Autodesk Inventor part; units mm, degrees
ref_plane "YZ Plane" through (0, 0, 0) normal (1, 0, 0) x (0, 1, 0)
ref_plane "XZ Plane" through (0, 0, 0) normal (0, 1, 0) x (-1, 0, 0)
ref_plane "XY Plane" through (0, 0, 0) normal (0, 0, 1) x (1, 0, 0)
sketch "Sketch1" plane through (0, 0, 0) normal (0, 1, 0) x (-1, 0, 0)
  line L0 (0, -74.6125) -> (0, -76.2)
  line L1 (0, -76.2) -> (-1.461, -76.8211)
  line L2 (-70.1269, -106.0104) -> (-75.0953, -94.3226)
  line L3 (0, 0) -> (-12.7, 0)
  line L4 (0, 0) -> (12.7, 0)
  line L5 (-75.0953, -94.3226) -> (-12.7, -67.7988)
  line L6 (-12.7, 0) -> (-12.7, -67.7988)
  line L7 (-70.1269, -106.0104) -> (-65.1585, -117.6982)
  line L8 (-65.1585, -117.6982) -> (12.7, -84.6012)
  line L9 (12.7, -84.6012) -> (12.7, 0)
  circle A0 centre (0, -76.2) radius 1.5875
  dimension "d0" = 76.2
  dimension "d1" = 76.2
  dimension "d2" = 113.03
  dimension "d3" = 12.7
  dimension "d4" = 12.7
  dimension "d5" = 12.7
  dimension "d6" = 12.7
  dimension "d7" = 3.175
extrude "Extrusion1" add sketch "Sketch1" along normal blind 6.35
sketch "Sketch2" plane through (-12.7, 0, 0) normal (0, 0, 1) x (1, 0, 0)
  circle A0 centre (12.7, 3.175) radius 1.5875
  point P0 (12.7, 0)
  dimension "d10" = 3.175
extrude "Extrusion2" cut sketch "Sketch2" against normal blind 19.05
sketch "Sketch3" plane through (65.1585, 0, -117.6982) normal (0.9203001, 0, -0.3912131) x (-0.3912131, 0, -0.9203001)
  circle A0 centre (-12.7, 3.175) radius 1.5875
  point P0 (-82.8269, 0)
  dimension "d13" = 3.175
extrude "Extrusion3" cut sketch "Sketch3" against normal blind 19.05
fillet "Fillet1" radius 6.35 1 edges at (-12.7, 3.175, -84.6012)
fillet "Fillet2" radius 6.35 1 edges at (12.7, 3.175, -67.7988)
fillet "Fillet3" radius 6.35 1 edges at (65.1585, 3.175, -117.6982)
fillet "Fillet4" radius 6.35 1 edges at (75.0953, 3.175, -94.3226)
fillet "Fillet5" radius 6.35 1 edges at (12.7, 3.175, 0)
fillet "Fillet6" radius 6.35 1 edges at (-12.7, 3.175, 0)
sketch "Sketch4" plane through (0, 6.35, 0) normal (0, 1, 0) x (1, 0, 0)
  circle A0 centre (0, 76.2) radius 1.5875
  circle A1 centre (0, 76.2) radius 3.175
  point P0 (0, 0)
  dimension "d22" = 6.35
extrude "Extrusion4" cut sketch "Sketch4" against normal blind 1.5875
sketch "Sketch5" plane through (0, 6.35, 0) normal (0, 1, 0) x (1, 0, 0)
  arc A0 (69.2514, 91.8384) -> (72.6111, 100.1665) centre (66.7672, 97.6823) ccw
  circle A1 centre (66.7672, 97.6823) radius 1.5875
  point P0 (0, 0)
  dimension "d25" = 3.175
extrude "Extrusion5" cut sketch "Sketch5" against normal blind 6.35
sketch "Sketch6" plane through (0, 0, 0) normal (0, -1, 0) x (1, 0, 0)
  circle A0 centre (66.7672, -97.6823) radius 1.5875
  arc A1 (72.6111, -100.1665) -> (69.2514, -91.8384) centre (66.7672, -97.6823) ccw
  circle A2 centre (66.7672, -97.6823) radius 3.175
  point P0 (0, 0)
  dimension "d28" = 6.35
extrude "Extrusion6" cut sketch "Sketch6" against normal blind 1.5875
sketch "Sketch7" plane through (0, 0, 0) normal (0, -1, 0) x (1, 0, 0)
  arc A0 (12.7, -6.35) -> (6.35, 0) centre (6.35, -6.35) ccw
  circle A1 centre (6.35, -6.35) radius 1.5875
  point P0 (0, 0)
  dimension "d31" = 3.175
extrude "Extrusion7" cut sketch "Sketch7" against normal blind 6.35
sketch "Sketch8" plane through (0, 0, 0) normal (0, -1, 0) x (1, 0, 0)
  circle A0 centre (6.35, -6.35) radius 1.5875
  arc A1 (12.7, -6.35) -> (6.35, 0) centre (6.35, -6.35) ccw
  circle A2 centre (6.35, -6.35) radius 3.175
  point P0 (0, 0)
  dimension "d34" = 6.35
extrude "Extrusion8" cut sketch "Sketch8" against normal blind 1.5875
sketch "Sketch9" plane through (0, 3.175, -19.05) normal (0, 0, 1) x (1, 0, 0)
  circle A0 centre (0, 0) radius 1.5875
  point P0 (0, -3.175)
extrude "Extrusion9" cut sketch "Sketch9" against normal blind 31.75
sketch "Sketch10" plane through (52.5952, 3.175, -98.5578) normal (0.9203001, 0, -0.3912131) x (-0.3912131, 0, -0.9203001)
  circle A0 centre (0, 0) radius 1.5875
  point P0 (-70.1269, -3.175)
extrude "Extrusion10" cut sketch "Sketch10" against normal blind 31.75
sketch "Sketch11" plane through (0, 6.35, 0) normal (0, 1, 0) x (1, 0, 0)
  line L0 (-12.7, 80.4006) -> (-12.7, 6.35)
  line L1 (0, 57.15) -> (6.35, 57.15)
  line L2 (6.35, 57.15) -> (6.35, 44.45)
  line L3 (6.35, 44.45) -> (-6.35, 44.45)
  line L4 (-6.35, 44.45) -> (-6.35, 57.15)
  line L5 (-6.35, 57.15) -> (0, 57.15)
  point P0 (0, 0)
  dimension "d41" = 6.35
  dimension "d42" = 12.7
  dimension "d43" = 12.7
  dimension "d44" = 12.7
extrude "Extrusion11" cut sketch "Sketch11" against normal blind 31.75
sketch "Sketch12" plane through (0, 6.35, 0) normal (0, 1, 0) x (1, 0, 0)
  line L0 (72.6111, 100.1665) -> (67.6427, 111.8543)
  line L1 (59.3146, 115.214) -> (-8.8342, 86.2445)
  line L2 (29.2195, 88.621) -> (17.5317, 83.6526)
  line L3 (17.5317, 83.6526) -> (15.0475, 89.4965)
  line L4 (15.0475, 89.4965) -> (26.7353, 94.4649)
  line L5 (26.7353, 94.4649) -> (31.7037, 82.7771)
  line L6 (31.7037, 82.7771) -> (20.0159, 77.8087)
  line L7 (20.0159, 77.8087) -> (17.5317, 83.6526)
  point P0 (0, 0)
  point P1 (70.1269, 106.0104)
  dimension "d47" = 57.15
  dimension "d48" = 6.35
  dimension "d49" = 12.7
  dimension "d50" = 12.7
  dimension "d51" = 12.7
extrude "Extrusion12" cut sketch "Sketch12" against normal blind 31.75 contours L5 L6 L7 L2
sketch "Sketch13" plane through (0, 6.35, 0) normal (0, 1, 0) x (1, 0, 0)
  line L0 (17.5317, 83.6526) -> (29.2195, 88.621)
  line L1 (59.3146, 115.214) -> (-8.8342, 86.2445)
  line L2 (17.5317, 83.6526) -> (15.0475, 89.4965)
  line L3 (15.0475, 89.4965) -> (26.7353, 94.4649)
  line L4 (26.7353, 94.4649) -> (29.2195, 88.621)
  point P0 (0, 0)
  dimension "d54" = 6.35
  dimension "d55" = 12.7
extrude "Extrusion13" cut sketch "Sketch13" against normal blind 31.75
sketch "Sketch14" plane through (6.35, 0, 0) normal (0, 0, 1) x (1, 0, 0)
  circle A0 centre (-6.35, 3.175) radius 1.5875
  circle A1 centre (-6.35, 3.175) radius 2.286
  point P0 (-6.35, 0)
  dimension "d58" = 4.572
extrude "Extrusion14" cut sketch "Sketch14" against normal blind 44.45
sketch "Sketch15" plane through (67.6427, 0, -111.8543) normal (0.9203001, 0, -0.3912131) x (-0.3912131, 0, -0.9203001)
  circle A0 centre (-6.35, 3.175) radius 1.5875
  circle A1 centre (-6.35, 3.175) radius 2.286
  point P0 (-76.4769, 0)
  dimension "d61" = 4.572
extrude "Extrusion15" cut sketch "Sketch15" against normal blind 44.45
sketch "Sketch16" plane through (0, 6.35, 0) normal (0, 1, 0) x (1, 0, 0)
  circle A0 centre (0, 76.2) radius 3.175
  line L0 (59.3146, 115.214) -> (-8.8342, 86.2445)
  arc A1 (-8.8342, 86.2445) -> (-12.7, 80.4006) centre (-6.35, 80.4006) ccw
  line L1 (-12.7, 80.4006) -> (-12.7, 6.35)
  line L2 (-31.4662, 97.6823) -> (-24.3054, 108.171)
  line L3 (-24.3054, 108.171) -> (1.4241, 90.6052)
  line L4 (-31.4662, 97.6823) -> (-38.6269, 87.1936)
  line L5 (-38.6269, 87.1936) -> (-12.7, 69.493)
  line L6 (0, 76.2) -> (-2.6222, 77.9902)
  point P0 (0, 0)
  dimension "d64" = 38.1
  dimension "d65" = 12.7
  dimension "d66" = 12.7
extrude "Extrusion16" add sketch "Sketch16" against normal blind 6.35 contours L0 A1 L1 L5 L4 L2 L3
sketch "Sketch17" plane through (0, 6.35, 0) normal (0, 1, 0) x (1, 0, 0)
  line L0 (-24.3054, 108.171) -> (-38.6269, 87.1936)
  line L1 (-38.6269, 87.1936) -> (-12.7, 69.493)
  line L2 (-31.4662, 97.6823) -> (-23.5996, 92.3117)
  circle A0 centre (-23.5996, 92.3117) radius 1.5875
  point P0 (0, 0)
  dimension "d69" = 9.525
  dimension "d70" = 3.175
extrude "Extrusion17" cut sketch "Sketch17" against normal blind 6.35
sketch "Sketch18" plane through (0, 6.35, 0) normal (0, 1, 0) x (1, 0, 0)
  circle A0 centre (-23.5996, 92.3117) radius 1.5875
  line L0 (26.7353, 94.4649) -> (31.7037, 82.7771)
  line L1 (31.7037, 82.7771) -> (20.0159, 77.8087)
  line L2 (20.0159, 77.8087) -> (15.0475, 89.4965)
  line L3 (15.0475, 89.4965) -> (26.7353, 94.4649)
  line L4 (-6.35, 44.45) -> (-6.35, 57.15)
  line L5 (-6.35, 57.15) -> (6.35, 57.15)
  line L6 (6.35, 57.15) -> (6.35, 44.45)
  line L7 (6.35, 44.45) -> (-6.35, 44.45)
  circle A1 centre (6.35, 6.35) radius 1.5875
  circle A2 centre (66.7672, 97.6823) radius 1.5875
  circle A3 centre (0, 76.2) radius 3.175
  arc A4 (-12.7, 6.35) -> (-6.35, 0) centre (-6.35, 6.35) ccw
  line L8 (-6.35, 0) -> (6.35, 0)
  arc A5 (6.35, 0) -> (12.7, 6.35) centre (6.35, 6.35) ccw
  line L9 (12.7, 6.35) -> (12.7, 63.5983)
  arc A6 (16.5658, 69.4422) -> (12.7, 63.5983) centre (19.05, 63.5983) ccw
  line L10 (16.5658, 69.4422) -> (69.2514, 91.8384)
  arc A7 (69.2514, 91.8384) -> (72.6111, 100.1665) centre (66.7672, 97.6823) ccw
  line L11 (72.6111, 100.1665) -> (67.6427, 111.8543)
  arc A8 (67.6427, 111.8543) -> (59.3146, 115.214) centre (61.7988, 109.3701) ccw
  line L12 (59.3146, 115.214) -> (1.4241, 90.6052)
  line L13 (1.4241, 90.6052) -> (-24.3054, 108.171)
  line L14 (-24.3054, 108.171) -> (-38.6269, 87.1936)
  line L15 (-38.6269, 87.1936) -> (-12.7, 69.493)
  line L16 (-12.7, 69.493) -> (-12.7, 6.35)
  point P0 (0, 0)
sketch "Sketch19" plane through (0, 0, 0) normal (0, -1, 0) x (1, 0, 0)
  circle A0 centre (-23.5996, -92.3117) radius 1.5875
  circle A1 centre (-23.5996, -92.3117) radius 3.175
  point P0 (0, 0)
  dimension "d73" = 6.35
extrude "Extrusion18" cut sketch "Sketch19" against normal blind 1.5875
fillet "Fillet7" radius 6.35 1 edges at (-24.3054, 3.175, -108.171)
fillet "Fillet8" radius 6.35 1 edges at (-38.6269, 3.175, -87.1936)
fillet "Fillet9" radius 6.35 1 edges at (1.4241, 3.175, -90.6052)
fillet "Fillet10" radius 6.35 1 edges at (-12.7, 3.175, -69.493)
properties part number "Auto Steering Part"
For this review, take the finished solid that the model builds, in its own axes (mm). A direction names the side the tool comes from. Round coordinates to 2 decimals unless told otherwise and drop trailing zeros. Write each loop counter-clockwise with the first axis right and the second up, starting at its lowest first coordinate (ties: lowest second). Pieces come first, ordered by that corner, then holes. Notation, with made-up numbers: (-37.5, 65) - (20.5, 65) arc R33 ccw to (20.5, 94) - close; hole circle Ø4 at (73, 39.5). An arc over 180 degrees is marked (long way). Write item = value, one per line. Start each with the question number.
1. For faces 4 (the face through (-10.376, 3.219, -98.661)), 5 (the face through (1.707, 5.567, -78.877)), 6 (the face through (25.942, 3.219, -80.328)), list the 3-axis set-ups (+Z, -Z, +X, -X, +Y, -Y) from which the entire face can be reached by the end or side of a thin tool; tool diameter is ignored.
2. Draft analysis for pull direction X (two halves, no side actions). For faces 1 (the face through (14, 0, -71)), 2 (the face through (12.7, 3, -35)), 3 (the face through (-6.35, 3, -51)), state which applies: released by +X, released by -X, zero draft, split by the parting line, or undercut.
3. Consider section A-A on x = 0. Give the number of separate pieces and of enclosed holes in the cut face, plus the area to 3 significant figures.
4. Consider section D-D on z = -62. State the section outline as (x, y) points.
5. Wall thickness on L1, parallel to X at y = 1.75, z = -61; L2, parallel to Z at x = -5, y = 3.75; L3, parallel to X at y = 3.5, z = -101: over which ranges is each line inside the solid? List them lowest first.
6. Consider section B-B on z = -37.5. State the section outline as (x, y) points (3 decimals), plus the area to 3 significant figures.
7. For pin 1 Ø1.9 at (x, z) = (5.5, -5) entering from -Y; pin 2 Ø2 at (x, y) = (28, 1.5) entering from -Z; pin 3 Ø3 at (x, z) = (0.5, -77) entering from +Y, all flat-tipped, find the tip position at first contact; note any pin that passes through.
Evaluation:
q1.face_4 = -Z, +Y, -Y
q1.face_5 = +Y
q1.face_6 = +Y, -Y
q2.face_1 = zero draft
q2.face_2 = released by +X
q2.face_3 = undercut
q3.separate_pieces = 4
q3.enclosed_holes = 0
q3.area = 274 mm2
q4.outline = (-12.7, 0) - (12.7, 0) - (12.7, 6.35) - (-12.7, 6.35) - close
q5.L1 = -12.7 to 12.7
q5.L2 = -94.99 to -57.15, -44.45 to 0
q5.L3 = -29.2 to -13.8, 25.88 to 52.56, 64.12 to 72.26
q6.outline = (-12.7, 0) - (12.7, 0) - (12.7, 6.35) - (-12.7, 6.35) - close; hole circle Ø4.572 at (0, 3.175)
q6.area = 145 mm2
q7.pin_1 = 1.59
q7.pin_2 = -102.33
q7.pin_3 = 4.76
